Geometry: final body of the model. Coordinates: model frame, mm. A direction names the side the tool comes from. Give positions to 0.01 mm unless a question says otherwise; leave off trailing zeros. Loops run counter-clockwise (first coordinate to the right, second up) from the corner with the lowest first, then second, coordinate; pieces in that order, holes last.
1. Access query for faces 4 (the face through (-52.25, -24, 4)), 5 (the face through (-1, 38, 6)), 6 (the face through (52.25, -36, 9)), 7 (the face through (23, -34, 9)), 8 (the face through (-4.7, -36, 9)). Directions: +Z, -Z, +X, -X, +Y, -Y. A direction counts if a zero-diameter tool reaches every point of the face in a straight line with its end or side. Return the directions, or none.
2. Section C-C, the plane y = -5. State how many separate pieces and enclosed holes the cut face has, then the cut area to 4 significant figures.
3. Draft query along X for faces 1 (the face through (-54.28, -5.77, 54.04)), 2 (the face through (-39.973, -35.972, 8.912)), 3 (the face through (52.25, 36, 9)). Return one class per face: +X half, -X half, draft (parallel to the pull), parting line (faces both ways), or undercut.
4. First-contact query: P1, Ø4, axis at x = 82, y = -32, coming from the +Z side; P2, Ø3.5, axis at x = 57.75, y = 43.3, coming from the +Z side; P3, Ø6.5, axis at x = 9.575, z = 9, coming from the -Y side; P4, Ø3, axis at y = 35.5, z = 8, coming from the -X side. Flat tips, straight axial feed; report the tip coordinate or a pass-through.
5. Section B-B, the plane x = 4.5. Output: boundary loops of the cut face in (y, z).
6. Section D-D, the plane x = 57.75. Output: boundary loops of the cut face in (y, z).
7. Section A-A, the plane y = -50.8. Output: boundary loops of the cut face in (x, z).
8. Material intervals for line 1 along X through (y, z) = (-58, 3); line 2 along Y through (x, z) = (-31.5, 7); line 3 along X through (y, z) = (-4.5, 22.5), sorted ascending.
Autodesk Inventor part; units mm, degrees
ref_plane "YZ Plane" through (0, 0, 0) normal (1, 0, 0) x (0, 1, 0)
ref_plane "XZ Plane" through (0, 0, 0) normal (0, 1, 0) x (-1, 0, 0)
ref_plane "XY Plane" through (0, 0, 0) normal (0, 0, 1) x (1, 0, 0)
sketch "Эскиз1" plane through (0, 0, 0) normal (0, 0, 1) x (1, 0, 0)
  line L0 (-42.5, -28.25) -> (42.5, -28.25) construction
  line L1 (42.5, -28.25) -> (42.5, 28.25) construction
  line L2 (42.5, 28.25) -> (-42.5, 28.25) construction
  line L3 (-42.5, 28.25) -> (-42.5, -28.25) construction
  line L4 (-52.25, 38) -> (52.25, 38)
  line L5 (52.25, 38) -> (52.25, -38)
  line L6 (52.25, -38) -> (-52.25, -38)
  line L7 (-52.25, -38) -> (-52.25, 38)
  line L8 (52.25, 38) -> (52.25, 68) construction
  line L9 (52.25, 68) -> (105.25, 68) construction
  line L10 (105.25, 68) -> (105.25, 0) construction
  line L11 (105.25, 0) -> (105.25, -68) construction
  line L12 (105.25, -68) -> (52.25, -68) construction
  line L13 (52.25, -68) -> (52.25, 0) construction
  line L14 (52.25, 38) -> (52.25, 68)
  line L15 (105.25, 68) -> (52.25, 68)
  line L16 (105.25, 68) -> (105.25, -68)
  line L17 (105.25, -68) -> (52.25, -68)
  line L18 (52.25, -68) -> (52.25, 0)
  line L19 (-42.5, -28.25) -> (42.5, -28.25)
  line L20 (42.5, 28.25) -> (42.5, -28.25)
  line L21 (-42.5, -28.25) -> (-42.5, 28.25)
  line L22 (42.5, 28.25) -> (-42.5, 28.25)
  dimension "d0" = 85
  dimension "d1" = 56.5
  dimension "d2" = 9.75
  dimension "d3" = 68
  dimension "d4" = 53
  dimension "d5" = 68
extrude "Выдавливание1" add sketch "Эскиз1" along normal blind 5 contours L4 L5 L6 L7 | L14 L15 L16 L17 L18 L5 | L21 L22 L20 L19
sketch "Эскиз4" plane through (0, 0, 5) normal (0, 0, 1) x (1, 0, 0)
  line L0 (-42.5, -28.25) -> (42.5, -28.25) construction
  line L1 (-42.5, -28.25) -> (-42.5, 28.25)
  line L2 (42.5, 28.25) -> (-42.5, 28.25) construction
  line L3 (-42.5, 28.25) -> (42.5, 28.25)
  line L4 (42.5, 28.25) -> (42.5, -28.25)
  line L5 (42.5, -28.25) -> (-42.5, -28.25)
  line L6 (-42.5, -28.25) -> (-42.5, 28.25)
  point P0 (0, 0)
extrude "Выдавливание3" cut sketch "Эскиз4" against normal blind 1
sketch "Эскиз5" plane through (0, 0, 4) normal (0, 0, 1) x (1, 0, 0)
  line L0 (42.5, 28.25) -> (42.5, -28.25)
  line L1 (-42.5, 28.25) -> (42.5, 28.25)
  line L2 (-42.5, -28.25) -> (-42.5, 28.25)
  line L3 (42.5, -28.25) -> (-42.5, -28.25)
  line L4 (32.25, 18) -> (32.25, -18)
  line L5 (32.25, -18) -> (-32.25, -18)
  line L6 (-32.25, -18) -> (-32.25, 18)
  line L7 (-32.25, 18) -> (32.25, 18)
  point P0 (0, 0)
  dimension "d12" = 10.25
extrude "Выдавливание4" cut sketch "Эскиз5" against normal blind 8 contours L4 L5 L6 L7
sketch "Эскиз6" plane through (0, 0, 5) normal (0, 0, 1) x (1, 0, 0)
  line L0 (-33.05, 26.6205) -> (33.05, 26.6205) construction
  line L1 (33.05, 26.6205) -> (33.05, -26.6205) construction
  line L2 (33.05, -26.6205) -> (-33.05, -26.6205) construction
  line L3 (-33.05, -26.6205) -> (-33.05, 26.6205) construction
  line L4 (-33.05, 26.6205) -> (33.05, -26.6205) construction
  line L5 (33.05, 26.6205) -> (-33.05, -26.6205) construction
  point P0 (0, 0)
  dimension "d15" = 66.1
  dimension "d16" = 53.241
sketch "Эскиз7" plane through (0, 0, 5) normal (0, 0, 1) x (1, 0, 0)
  line L0 (-52.25, 38) -> (-52.25, -38) construction
  line L1 (-52.25, 0) -> (-56.25, 0)
  line L2 (-56.25, 10) -> (-52.25, 10)
  line L3 (-52.25, 10) -> (-52.25, -10)
  line L4 (-52.25, -10) -> (-56.25, -10)
  line L5 (-56.25, -10) -> (-56.25, 10)
  line L6 (-56.25, 10) -> (-52.25, -10) construction
  line L7 (-52.25, 10) -> (-56.25, -10) construction
  point P0 (0, 0)
  point P1 (-54.25, 0)
  dimension "d17" = 4
  dimension "d18" = 20
extrude "Выдавливание5" add sketch "Эскиз7" along normal blind 75 and the other way blind 5
sketch "Эскиз8" plane through (-56.25, -10, 80) normal (-1, 0, 0) x (0, 0, 1)
  line L0 (0, 0) -> (-80, 0)
  line L1 (0, 20) -> (0, 0)
  line L2 (-80, 20) -> (0, 20)
  line L3 (-80, 0) -> (-80, 20)
  line L4 (-80, 0) -> (-33.989, 0) construction
  line L5 (0, 0) -> (-80, 0) construction
  line L6 (-33.989, 0) -> (-33.989, 20) construction
  line L7 (0, 20) -> (-75, 20) construction
  line L8 (-33.989, 20) -> (-27.805, 20) construction
  line L9 (-27.805, 20) -> (-27.805, 14.454) construction
  circle A0 centre (-27.805, 14.454) radius 2
  line L10 (-27.805, 14.454) -> (-21.488, 14.454) construction
  line L11 (-27.805, 14.454) -> (-27.805, 5) construction
  circle A1 centre (-27.805, 5) radius 2
  circle A2 centre (-21.488, 14.454) radius 2
  circle A3 centre (-21.488, 5) radius 2
  circle A4 centre (-15.171, 14.454) radius 2
  circle A5 centre (-15.171, 5) radius 2
  circle A6 centre (-8.854, 14.454) radius 2
  circle A7 centre (-8.854, 5) radius 2
  point P0 (-80, 10)
  dimension "d23" = 46.011
  dimension "d24" = 6.184
  dimension "d25" = 5.546
  dimension "d26" = 4
  dimension "d27" = 6.317
  dimension "d28" = 9.454
  dimension "d29" = 4
  dimension "d32" = 6.317
extrude "Выдавливание6" cut sketch "Эскиз8" against normal blind 75 contours A0 | A1 | A2 | A3 | A4 | A5 | A6 | A7
sketch "Эскиз9" plane through (0, 0, 0) normal (0, 0, -1) x (-1, 0, 0)
  line L0 (-32.25, 18) -> (32.25, 18)
  line L1 (32.25, 18) -> (32.25, -18)
  line L2 (32.25, -18) -> (-32.25, -18)
  line L3 (-32.25, -18) -> (-32.25, 18)
  line L4 (-52.25, 68) -> (-52.25, 38)
  line L5 (-105.25, 68) -> (-52.25, 68)
  line L6 (-105.25, -68) -> (-105.25, 68)
  line L7 (-52.25, -68) -> (-105.25, -68)
  line L8 (-52.25, -38) -> (-52.25, -68)
  line L9 (52.25, -38) -> (-52.25, -38)
  line L10 (52.25, -10) -> (52.25, -38)
  line L11 (52.25, -10) -> (56.25, -10)
  line L12 (56.25, -10) -> (56.25, 10)
  line L13 (56.25, 10) -> (52.25, 10)
  line L14 (52.25, 38) -> (52.25, 10)
  line L15 (-52.25, 38) -> (52.25, 38)
  line L16 (52.25, -38) -> (52.25, -42) construction
  line L17 (52.25, -38) -> (-52.25, -38)
  line L18 (52.25, -38) -> (23.7, -38)
  line L19 (4.7, -38) -> (-23.85, -38)
  line L20 (56.25, 0) -> (0, 0) construction
  line L21 (52.25, 38) -> (-52.25, 38)
  line L22 (52.25, 38) -> (52.25, 42) construction
  line L23 (4.7, 38) -> (-23.85, 38)
  line L24 (23.7, 34) -> (52.25, 34)
  line L25 (23.7, 38) -> (23.7, 34)
  line L26 (52.25, 38) -> (52.25, 34) construction
  line L27 (52.25, 34) -> (52.25, 38)
  line L28 (4.7, 34) -> (4.7, 38)
  line L29 (-23.85, 34) -> (4.7, 34)
  line L30 (-23.85, 38) -> (-23.85, 34)
  line L31 (52.25, -38) -> (52.25, -34) construction
  line L32 (23.7, -38) -> (23.7, -34)
  line L33 (23.7, -34) -> (52.25, -34)
  line L34 (52.25, -34) -> (52.25, -38)
  line L35 (-23.85, -38) -> (-23.85, -34)
  line L36 (-23.85, -34) -> (4.7, -34)
  line L37 (4.7, -34) -> (4.7, -38)
  line L38 (52.25, 34) -> (23.7, 34)
  line L39 (23.7, 34) -> (23.7, 38)
  line L40 (23.7, 38) -> (52.25, 38)
  line L41 (52.25, 38) -> (52.25, 34)
  line L42 (4.7, 34) -> (-23.85, 34)
  line L43 (-23.85, 34) -> (-23.85, 38)
  line L44 (-23.85, 38) -> (4.7, 38)
  line L45 (4.7, 38) -> (4.7, 34)
  dimension "d39" = 4
extrude "Выдавливание7" add sketch "Эскиз9" against normal blind 13 contours L15 L28 L29 L30 | L15 L14 L24 L25 | L35 L36 L37 L9 | L32 L33 L10 L9
sketch "Эскиз10" plane through (-52.25, 38, 0) normal (0, 1, 0) x (1, 0, 0)
  line L0 (47.55, -5) -> (28.55, -5) construction
  line L1 (28.55, -5) -> (0, -5) construction
  line L2 (0, 0) -> (0, -13) construction
  line L3 (0, -5) -> (0, -13) construction
  line L4 (0, -13) -> (0, -5) construction
  circle A0 centre (14.275, -9) radius 2
  line L5 (38.05, -7) -> (38.05, -12) construction
  circle A1 centre (61.825, -9) radius 2
  point P0 (52.25, 0)
  dimension "d45" = 4
extrude "Выдавливание8" cut sketch "Эскиз10" against normal up to surface (76 mm away)
sketch "Эскиз11" plane through (0, 0, 5) normal (0, 0, 1) x (1, 0, 0)
  line L0 (-42.5, 28.25) -> (42.5, 28.25)
  line L1 (42.5, 28.25) -> (42.5, -28.25)
  line L2 (42.5, -28.25) -> (-42.5, -28.25)
  line L3 (-42.5, -28.25) -> (-42.5, 28.25)
  line L4 (-23.7, 38) -> (-23.7, 34)
  line L5 (-23.7, 34) -> (-52.25, 34)
  line L6 (-52.25, 34) -> (-52.25, 10)
  line L7 (-52.25, 10) -> (-52.25, -10)
  line L8 (-52.25, -10) -> (-52.25, -34)
  line L9 (-52.25, -34) -> (-23.7, -34)
  line L10 (-23.7, -34) -> (-23.7, -38)
  line L11 (-23.7, -38) -> (-4.7, -38)
  line L12 (-4.7, -38) -> (-4.7, -34)
  line L13 (-4.7, -34) -> (23.85, -34)
  line L14 (23.85, -34) -> (23.85, -38)
  line L15 (23.85, -38) -> (52.25, -38)
  line L16 (52.25, -38) -> (52.25, -68)
  line L17 (52.25, -68) -> (105.25, -68)
  line L18 (105.25, -68) -> (105.25, 68)
  line L19 (105.25, 68) -> (52.25, 68)
  line L20 (52.25, 68) -> (52.25, 38)
  line L21 (52.25, 38) -> (23.85, 38)
  line L22 (23.85, 38) -> (23.85, 34)
  line L23 (23.85, 34) -> (-4.7, 34)
  line L24 (-4.7, 34) -> (-4.7, 38)
  line L25 (-4.7, 38) -> (-23.7, 38)
  line L26 (52.25, -38) -> (52.25, -68)
  line L27 (52.25, -68) -> (57.75, -68)
  line L28 (52.25, -68) -> (105.25, -68)
  line L29 (57.75, -68) -> (57.75, -38) construction
  line L30 (23.85, -38) -> (52.25, -38)
  line L31 (57.75, -38) -> (52.25, -38) construction
  line L32 (57.75, -68) -> (57.75, -58.3)
  circle A0 centre (57.75, -58.3) radius 2
  line L33 (57.75, -58.3) -> (57.75, -50.8) construction
  circle A1 centre (57.75, -50.8) radius 2
  circle A2 centre (57.75, -43.3) radius 2
  line L34 (52.25, -68) -> (105.25, -68) construction
  line L35 (78.75, -68) -> (78.75, -28.25) construction
  circle A3 centre (99.75, -58.3) radius 2
  circle A4 centre (99.75, -50.8) radius 2
  circle A5 centre (99.75, -43.3) radius 2
  line L36 (105.25, -68) -> (105.25, 68) construction
  line L37 (105.25, 0) -> (77, 0) construction
  circle A6 centre (57.75, 58.3) radius 2
  circle A7 centre (57.75, 50.8) radius 2
  circle A8 centre (57.75, 43.3) radius 2
  circle A9 centre (99.75, 58.3) radius 2
  circle A10 centre (99.75, 50.8) radius 2
  circle A11 centre (99.75, 43.3) radius 2
  point P0 (0, 0)
  dimension "d48" = 5.5
  dimension "d49" = 9.7
  dimension "d50" = 4
  dimension "d51" = 7.5
  dimension "d54" = 7.5
extrude "Выдавливание9" cut sketch "Эскиз11" against normal blind 10 contours A0 | A1 | A2 | A3 | A4 | A5 | A6 | A7 | A8 | A9 | A10 | A11
ref_plane "РабПлоскость1" through (23.85, 34, 13) normal (1, 0, 0) x (0, -1, 0)
sketch "Эскиз12" plane through (0, 0, 5) normal (0, 0, 1) x (1, 0, 0)
  line L0 (23.85, -34) -> (23.85, -38)
  line L1 (52.25, -38) -> (52.25, -68)
  line L2 (23.85, -34) -> (52.25, -34)
  line L3 (52.25, -34) -> (52.25, -38)
  line L4 (52.25, -38) -> (23.85, -38)
  line L5 (23.85, -38) -> (23.85, -34)
  line L6 (23.85, 34) -> (23.85, 38)
  line L7 (23.85, 38) -> (52.25, 38)
  line L8 (52.25, 38) -> (52.25, 34)
  line L9 (52.25, 34) -> (23.85, 34)
  line L10 (23.85, 34) -> (23.85, 38)
  point P0 (0, 0)
extrude "Выдавливание10" add sketch "Эскиз12" along normal up to surface (8 mm away)
sketch "Эскиз13" plane through (-52.25, -38, 0) normal (0, -1, 0) x (1, 0, 0)
  line L0 (47.55, 13) -> (104.5, 13)
  line L1 (76.025, 13) -> (76.025, 5)
  line L2 (9.75, 5) -> (94.75, 5)
  line L3 (157.5, 5) -> (104.5, 5)
  line L4 (76.025, 5) -> (104.5, 5)
  circle A0 centre (90.2625, 9) radius 2
  point P0 (52.25, 0)
  dimension "d63" = 4
extrude "Выдавливание11" cut sketch "Эскиз13" against normal up to surface (76 mm away)
properties part number "LIner"
Answers below:
1. face 4: +Z, -Z, -X, -Y
1. face 5: +Z, -Z, -X, +Y
1. face 6: +Z, +X, +Y, -Y
1. face 7: +Z, +X, -X
1. face 8: +Z, +Y, -Y
2. separate pieces: 6
2. enclosed holes: 0
2. area: 700.5 mm2
3. face 1: draft
3. face 2: undercut
3. face 3: +X half
4. P1: stops at z = 5
4. P2: passes through
4. P3: stops at y = -38
4. P4: stops at x = -52.25
5. outline: (-38, 0) - (-18, 0) - (-18, 4) - (-28.25, 4) - (-28.25, 5) - (-34, 5) - (-34, 13) - (-38, 13) - close; (18, 0) - (38, 0) - (38, 13) - (34, 13) - (34, 5) - (28.25, 5) - (28.25, 4) - (18, 4) - close
6. outline: (-68, 0) - (-60.3, 0) - (-60.3, 5) - (-68, 5) - close; (-56.3, 0) - (-52.8, 0) - (-52.8, 5) - (-56.3, 5) - close; (-48.8, 0) - (-45.3, 0) - (-45.3, 5) - (-48.8, 5) - close; (-41.3, 0) - (41.3, 0) - (41.3, 5) - (-41.3, 5) - close; (45.3, 0) - (48.8, 0) - (48.8, 5) - (45.3, 5) - close; (52.8, 0) - (56.3, 0) - (56.3, 5) - (52.8, 5) - close; (60.3, 0) - (68, 0) - (68, 5) - (60.3, 5) - close
7. outline: (52.25, 0) - (55.75, 0) - (55.75, 5) - (52.25, 5) - close; (59.75, 0) - (97.75, 0) - (97.75, 5) - (59.75, 5) - close; (101.75, 0) - (105.25, 0) - (105.25, 5) - (101.75, 5) - close
8. line 1: x = 52.25 to 55.77, 59.73 to 97.77, 101.73 to 105.25
8. line 2: y = -38 to -34, 34 to 38
8. line 3: x = -56.25 to -52.25
